Autodesk Inventor part; units mm, degrees
ref_plane "YZ Plane" through (0, 0, 0) normal (1, 0, 0) x (0, 1, 0)
ref_plane "XZ Plane" through (0, 0, 0) normal (0, 1, 0) x (-1, 0, 0)
ref_plane "XY Plane" through (0, 0, 0) normal (0, 0, 1) x (1, 0, 0)
sketch "Sketch1" plane through (0, 0, 0) normal (0, 1, 0) x (-1, 0, 0)
  line L0 (0, 0) -> (-15, 0)
  line L1 (-15, 0) -> (-15, 15)
  line L2 (-15, 15) -> (0, 15)
  line L3 (0, 15) -> (0, 0)
  line L4 (0, 0) -> (-2.5, 0)
  line L5 (-2.5, 0) -> (-2.5, 2.5)
  line L6 (-2.5, 2.5) -> (0, 2.5)
  line L7 (0, 2.5) -> (0, 0)
  line L8 (-2.5, 2.5) -> (-12.5, 2.5)
  line L9 (-12.5, 2.5) -> (-12.5, 12.5)
  line L10 (-12.5, 12.5) -> (-2.5, 12.5)
  line L11 (-2.5, 12.5) -> (-2.5, 2.5)
  dimension "d0" = 15
  dimension "d1" = 15
  dimension "d2" = 2.5
  dimension "d3" = 2.5
  dimension "d4" = 10
  dimension "d5" = 10
extrude "Extrusion1" add sketch "Sketch1" along normal blind 10
sketch "Sketch2" plane through (15, 0, 15) normal (1, 0, 0) x (0, 0, -1)
  line L0 (15, 0) -> (15, 10)
  line L1 (0, 10) -> (15, 10)
  line L2 (15, 10) -> (15, 0)
  line L3 (15, 0) -> (0, 0)
  line L4 (0, 0) -> (0, 10)
  line L5 (0, 0) -> (0, 10)
  line L6 (0, 10) -> (7.5, 10)
  line L7 (7.5, 10) -> (7.5, 5)
  line L8 (7.5, 5) -> (0, 5)
  line L9 (0, 5) -> (0, 10)
  circle A0 centre (7.5, 5) radius 1.4
  dimension "d8" = 7.5
  dimension "d9" = 5
  dimension "d10" = 2.8
extrude "Extrusion2" cut sketch "Sketch2" against normal through all contours A0 L8 L7 | L7 L8 A0
sketch "Sketch3" plane through (0, 0, 15) normal (0, 0, 1) x (1, 0, 0)
  line L0 (15, 10) -> (0, 10)
  line L1 (15, 0) -> (0, 0)
  line L2 (0, 10) -> (15, 10)
  line L3 (15, 10) -> (15, 0)
  line L4 (15, 0) -> (0, 0)
  line L5 (0, 0) -> (0, 10)
  line L6 (0, 10) -> (5, 10)
  line L7 (5, 10) -> (5, 7.5)
  line L8 (5, 7.5) -> (0, 7.5)
  line L9 (0, 7.5) -> (0, 10)
  line L10 (5, 7.5) -> (10, 7.5)
  line L11 (10, 7.5) -> (10, 2.5)
  line L12 (10, 2.5) -> (5, 2.5)
  line L13 (5, 2.5) -> (5, 7.5)
  dimension "d13" = 5
  dimension "d14" = 2.5
  dimension "d15" = 5
  dimension "d16" = 5
extrude "Extrusion3" add sketch "Sketch3" along normal blind 50 contours L10 L11 L12 L13
properties part number "CAM02"
Geometry check sheet. Reference: the model listing, model coordinates, mm. A direction names the side the tool comes from. Give positions to 0.01 mm unless a question says otherwise; leave off trailing zeros. Order: outer loops, then holes, each group sorted by start corner. A loop starts at its lowest first (then second) coordinate and runs counter-clockwise, first axis right, second up. Notation, with made-up numbers: (87.25, 11.25) -> (132.25, 11.25) arc R11 cw to (132.25, 22.25) -> close; hole circle Ø7 at (14, 65.5). An arc over 180 degrees is marked (long way). Write each question's results on one line, items separated by ' | '. Start each with the question number.
(1) Sectioned sample at B-B (z = 7.5). Enter the section's corners in (x, y).
(2) Access from +Z, -Z, +X, -X, +Y, -Y to the whole of each face (thin tool, end or side, straight path). Record for faces 1 (the face through (5, 5, 40)), 2 (the face through (12.5, 4, 6)), 3 (the face through (10, 5, 40)), 4 (the face through (0, 4.9, 9.3)), 5 (the face through (8, 2.5, 40)).
(3) Scan lines: line 1 (Y direction, x = 13.7, z = 7.5); line 2 (Z direction, x = 3.5, y = 7.25); line 3 (Z direction, x = 7.5, y = 4.5). Record each from-to range of solid material in increasing order.
(4) Sectioned sample at A-A (x = 7.75). Enter the section's corners in (y, z).
(5) Gauge pin test, flat ends, axial feed: P1, Ø4, axis at y = 4, z = 47.5, coming from the +X side; P2, Ø1.5, axis at x = 9.5, z = 20.5, coming from the -Y side; P3, Ø4, axis at x = 6.5, z = 41, coming from the +Y side. Record the tip position at first contact, or that the pin passes through.
(6) Sectioned sample at D-D (y = 1.75). Enter the section's corners in (x, z).
(7) Mould release check, pull along Z, two halves, no side actions. Record for faces 6 (the face through (7, 7.5, 40)), 7 (the face through (7, 5, 2.5)), 8 (the face through (7, 5, 0)): pulls with the +Z half, pulls with the -Z half, needs draft (parallel to the pull), parting line crosses it, or undercut.
(8) Sectioned sample at C-C (y = 5). Enter the section's corners in (x, z), plus the area to 3 significant figures.
Answer below:
1) outline: (0, 0) -> (2.5, 0) -> (2.5, 3.6) -> (0, 3.6) -> close; (0, 6.4) -> (2.5, 6.4) -> (2.5, 10) -> (0, 10) -> close; (12.5, 0) -> (15, 0) -> (15, 3.6) -> (12.5, 3.6) -> close; (12.5, 6.4) -> (15, 6.4) -> (15, 10) -> (12.5, 10) -> close
2) face 1: +Z, -X, +Y, -Y | face 2: +Y, -Y | face 3: +Z, +X, +Y, -Y | face 4: +Z, -Z, -X, +Y, -Y | face 5: +Z, +X, -X, -Y
3) line 1: 0 to 3.6, 6.4 to 10 | line 2: 0 to 2.5, 12.5 to 15 | line 3: 0 to 2.5, 12.5 to 65
4) outline: (0, 0) -> (10, 0) -> (10, 2.5) -> (0, 2.5) -> close; (0, 12.5) -> (10, 12.5) -> (10, 15) -> (7.5, 15) -> (7.5, 65) -> (2.5, 65) -> (2.5, 15) -> (0, 15) -> close
5) P1: x = 10 | P2: y = 2.5 | P3: y = 7.5
6) outline: (0, 0) -> (15, 0) -> (15, 15) -> (0, 15) -> close; hole (2.5, 2.5) -> (12.5, 2.5) -> (12.5, 12.5) -> (2.5, 12.5) -> close
7) face 6: needs draft | face 7: undercut | face 8: pulls with the -Z half
8) outline: (0, 0) -> (15, 0) -> (15, 6.1) -> (12.5, 6.1) -> (12.5, 2.5) -> (2.5, 2.5) -> (2.5, 6.1) -> (0, 6.1) -> close; (0, 8.9) -> (2.5, 8.9) -> (2.5, 12.5) -> (12.5, 12.5) -> (12.5, 8.9) -> (15, 8.9) -> (15, 15) -> (10, 15) -> (10, 65) -> (5, 65) -> (5, 15) -> (0, 15) -> close | area: 361 mm2
